Geometry: final body of the model. Coordinates: model frame, mm. Give positions to 0.01 mm unless a question says otherwise; leave off trailing zeros. Write each loop counter-clockwise with the first axis right and the second up, starting at its lowest first coordinate (ties: lowest second). Pieces come first, ordered by that corner, then holes. Notation, with made-up numbers: (50, 5.5) -> (78, 5.5) arc R26 cw to (78, 43.5) -> close; hole circle Ø9 at (-17.5, -26.75). An arc over 180 degrees is marked (long way). Answer in a Markdown table with one row per item. Add a question column.
Item 1: Material intervals for probe 1 along Y at (x, z) = (34.5, 0.8); probe 2 along X at (y, z) = (35.5, 1), sorted ascending. Write a range as from..to.
Item 2: Section query B-B on y = 45.5. Output: boundary loops of the cut face in (x, z), plus the area to 3 significant figures.
Item 3: Section query C-C on z = 0.55. Output: boundary loops of the cut face in (x, y), plus the area to 3 significant figures.
Item 4: Section query A-A on x = 30. Output: boundary loops of the cut face in (y, z), plus the area to 3 significant figures.
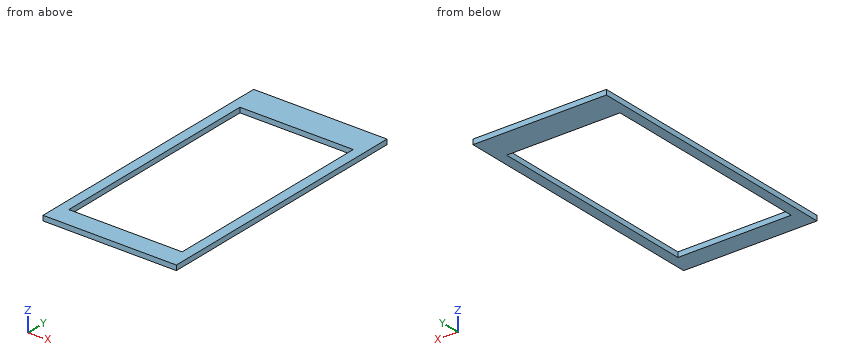
```python
from build123d import *

# Parameters (mm, degrees)
SKETCH1_W           = 40
SKETCH1_H           = 80
BOSS_EXTRUDE1_DEPTH = 1.5
CUT_EXTRUDE1_DEPTH  = 1.5


with BuildPart() as part:
    # Sketch1 → Boss-Extrude1 (new body)
    with BuildSketch(Plane.XY):
        with Locations((20, 40)):
            Rectangle(SKETCH1_W, SKETCH1_H)
    extrude(amount=BOSS_EXTRUDE1_DEPTH)

    # Sketch2 → Cut-Extrude1 (cut)
    with BuildSketch(Plane.XY.offset(1.5)):
        Polygon((37, 71), (37, 6), (20, 6), (3, 6), (3, 71), align=None)
    extrude(amount=-CUT_EXTRUDE1_DEPTH, mode=Mode.SUBTRACT)


solid = part.part
```
Findings below:
| question | item | result |
|---|---|---|
| 1 | probe 1 | y = 0..6, 71..80 |
| 1 | probe 2 | x = 0..3, 37..40 |
| 2 | outline | (0, 0) -> (3, 0) -> (3, 1.5) -> (0, 1.5) -> close; (37, 0) -> (40, 0) -> (40, 1.5) -> (37, 1.5) -> close |
| 2 | area | 9.00 mm^2 |
| 3 | outline | (0, 0) -> (40, 0) -> (40, 80) -> (0, 80) -> close; hole (3, 6) -> (37, 6) -> (37, 71) -> (3, 71) -> close |
| 3 | area | 990 mm^2 |
| 4 | outline | (0, 0) -> (6, 0) -> (6, 1.5) -> (0, 1.5) -> close; (71, 0) -> (80, 0) -> (80, 1.5) -> (71, 1.5) -> close |
| 4 | area | 22.5 mm^2 |
